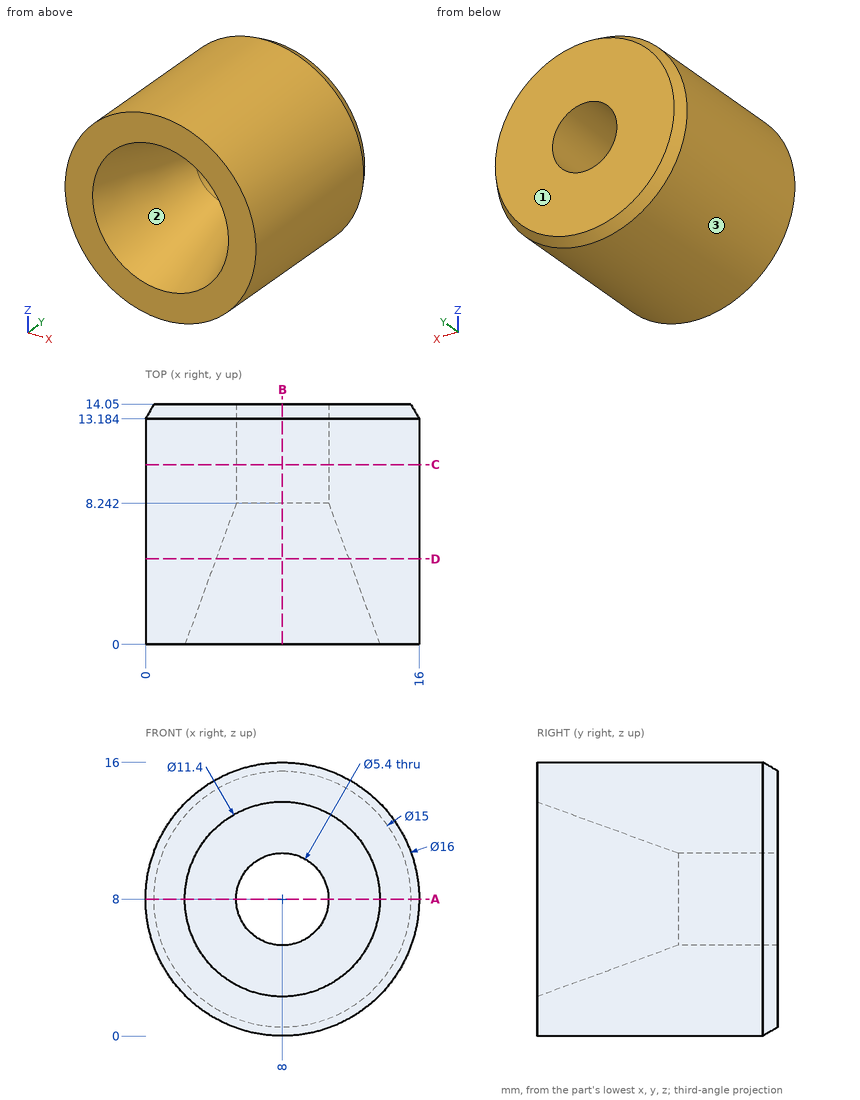
Geometry: see drawing. Coordinates: mm, zero at the bounding-box minimum. Give positions to 0.01 mm unless a question says otherwise; leave off trailing zeros. Order: outer loops, then holes, each group sorted by start corner. A loop starts at its lowest first (then second) coordinate and runs counter-clockwise, first axis right, second up.
Q1. Draft query along Z for the marked faces 1, 2 and 3. Return one class per face: +Z half, -Z half, draft (parallel to the pull), parting line (faces both ways), or undercut.
Checked values:
face 1: draft
face 2: undercut
face 3: parting line
Q2. Ray query, probe 1 along X at (y, z) = (12.15, 8); probe 2 along X at (y, z) = (9.25, 9); probe 3 along Z at (x, y) = (4.5, 4) (1 decimal). Return the intervals inside material, ascending.
Checked values:
probe 1: x = 0 to 5.3, 10.7 to 16
probe 2: x = 0.06 to 5.49, 10.51 to 15.94
probe 3: z = 0.8 to 5.6, 10.4 to 15.2
Q3. Section C-C on y = 10.5. Output: boundary loops of the cut face in (x, z).
Checked values:
outline: circle Ø16 at (8, 8); hole circle Ø5.4 at (8, 8)
Q4. Section A-A on z = 8. Output: boundary loops of the cut face in (x, y), and give its area (3 significant figures).
Checked values:
outline: (0, 0) - (2.3, 0) - (5.3, 8.24) - (5.3, 14.05) - (0.5, 14.05) - (0, 13.18) - close; (10.7, 8.24) - (13.7, 0) - (16, 0) - (16, 13.18) - (15.5, 14.05) - (10.7, 14.05) - close
area: 124 mm2
Q5. Section D-D on y = 5. Output: boundary loops of the cut face in (x, z), and give its area (3 significant figures).
Checked values:
outline: circle Ø16 at (8, 8); hole circle Ø7.76 at (8, 8)
area: 154 mm2
Q6. Contact query for flat-ended pins moving along their axis: pin 1 Ø5 at (x, y) = (4, 10.5) entering from +Z; pin 2 Ø3 at (x, z) = (8, 8) entering from -Y (1 decimal); pin 3 Ø4 at (y, z) = (3, 4) entering from +X; pin 4 Ø6 at (y, z) = (3.5, 7.5) entering from +X. Output: stop coordinate, or through.
Checked values:
pin 1: stops at z = 15.86
pin 2: passes through
pin 3: stops at x = 15.75
pin 4: stops at x = 16
Q7. Section B-B on x = 8. Output: boundary loops of the cut face in (y, z), and give its area (3 significant figures).
Checked values:
outline: (0, 0) - (13.18, 0) - (14.05, 0.5) - (14.05, 5.3) - (8.24, 5.3) - (0, 2.3) - close; (0, 13.7) - (8.24, 10.7) - (14.05, 10.7) - (14.05, 15.5) - (13.18, 16) - (0, 16) - close
area: 124 mm2
